Geometry check sheet. Reference: the model listing, model coordinates, mm. Face numbers are marked on the shaded views. A direction names the side the tool comes from. Round coordinates to 2 decimals unless told otherwise and drop trailing zeros. Write each loop counter-clockwise with the first axis right and the second up, starting at its lowest first coordinate (ties: lowest second). Pieces come first, ordered by that corner, then holes. Notation, with made-up numbers: M -2.5,-3.75 L 17.5,-3.75 A9 cw 17.5,3.25 Z; hole C 7.25,13 d6. An arc over 180 degrees is marked long. One line per item, written item: value. Start each with the question number.
1. Section check C-C (x = 0). Record the boundary of the cut face in (y, z).
2. Section check D-D (z = -11). Record the boundary of the cut face in (x, y), and give its area (3 significant figures).
3. Scan lines: probe 1 along Z at (x, y) = (0, 0.4); probe 2 along Y at (x, z) = (0, -6); probe 3 along X at (y, z) = (-17.5, 3). Record each from-to range of solid material in increasing order. Write a range as [from, to].
4. Release check for a two-part mould opening along X. For the marked faces 3, 4, 5 and 6 record: pulls with the +X half, pulls with the -X half, needs draft (parallel to the pull), parting line crosses it, or undercut.
5. Section check A-A (z = -16.5). Record the boundary of the cut face in (x, y).
6. Depth check by flat-ended pin: P1, Ø1.6, axis at y = 0.5, z = 20, coming from the +X side; P2, Ø1.5, axis at y = -20.5, z = 2.5, coming from the -X side; P3, Ø1.2, axis at x = 7.5, z = -4.5, coming from the -Y side. Enter the tip coordinate at first touch or a pass-through.
7. Section check B-B (y = -8.75). Record the boundary of the cut face in (x, z), and give its area (3 significant figures).
8. Access from +Z, -Z, +X, -X, +Y, -Y to the whole of each face (thin tool, end or side, straight path). Record for the marked faces 1 and 2.
Autodesk Inventor part; units mm, degrees
ref_plane "YZ Plane" through (0, 0, 0) normal (1, 0, 0) x (0, 1, 0)
ref_plane "XZ Plane" through (0, 0, 0) normal (0, 1, 0) x (-1, 0, 0)
ref_plane "XY Plane" through (0, 0, 0) normal (0, 0, 1) x (1, 0, 0)
sketch "Sketch1" plane through (0, 0, 0) normal (0, 1, 0) x (-1, 0, 0)
  line L0 (5, 25) -> (-5, 25)
  line L1 (-5, 25) -> (-5, -25)
  line L2 (-5, -25) -> (5, -25)
  line L3 (5, -25) -> (5, 25)
  line L4 (5, 25) -> (-5, -25) construction
  line L5 (-5, 25) -> (5, -25) construction
  circle A0 centre (0, 15) radius 2.5
  circle A1 centre (0, -15) radius 2.5
  point P0 (0, 0)
  point P1 (0, 25)
  dimension "d0" = 10
  dimension "d1" = 50
  dimension "d2" = 5
  dimension "d3" = 5
  dimension "d4" = 30
  dimension "d5" = 10
  dimension "d6" = 5
  dimension "d7" = 5
extrude "Extrusion1" add sketch "Sketch1" along normal blind 2
sketch "Sketch2" plane through (0, 0, 0) normal (0, -1, 0) x (1, 0, 0)
  line L0 (-5, -15) -> (-9, -15)
  line L1 (-5, 15) -> (-5.5, 15)
  circle A0 centre (0, -15) radius 2.5
  circle A1 centre (0, 15) radius 2.5
  arc A2 (-5.5, 15) -> (-9, -15) centre (110.994, -13.7951) ccw
  line L2 (-5, -15) -> (-5, 15)
  line L3 (-5, -25) -> (-5, 25)
  point P0 (0, 0)
  point P1 (-4, -14.9499)
  point P2 (-3, -15)
  dimension "d10" = 0
  dimension "d11" = 0
  dimension "d12" = 4
  dimension "d13" = 0.5
  dimension "d14" = 120
  dimension "d15" = 0
  dimension "d16" = 0
  dimension "d17" = 0
extrude "Extrusion2" add sketch "Sketch2" along normal blind 25 and the other way blind 2 contours L0 A2 L1 L2
sketch "Sketch3" plane through (0, 2, 0) normal (0, 1, 0) x (1, 0, 0)
  line L0 (5, -25) -> (5, 25)
  line L1 (5, 15) -> (9, 15)
  line L2 (5, -15) -> (5.5, -15)
  line L3 (5, -15) -> (5, 15)
  circle A0 centre (0, 15) radius 2.5
  circle A1 centre (0, -15) radius 2.5
  arc A2 (5.5, -15) -> (9, 15) centre (-110.994, 13.7951) ccw
  point P0 (0, 0)
  dimension "d22" = 0
  dimension "d23" = 0
  dimension "d24" = 0.5
  dimension "d25" = 4
  dimension "d26" = 120
extrude "Extrusion3" add sketch "Sketch3" against normal blind 25 contours L0 L1 A2 L2
properties part number "squeezer"
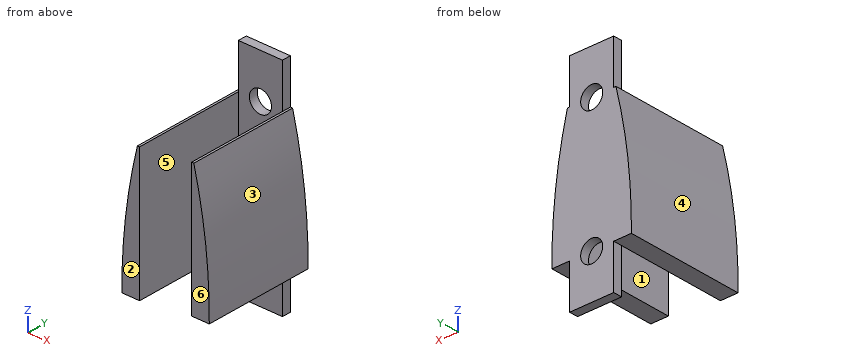
Result sheet:
1. outline: M 0,-25 L 2,-25 L 2,-17.5 L 0,-17.5 Z; M 0,-12.5 L 2,-12.5 L 2,12.5 L 0,12.5 Z; M 0,17.5 L 2,17.5 L 2,25 L 0,25 Z
2. outline: M -8.97,-25 L -5,-25 L -5,0 L 5,0 L 5,-23 L 8.97,-23 L 8.97,2 L -8.97,2 Z
2. area: 227 mm2
3. probe 1: z = [-25, -17.5], [-12.5, 12.5], [17.5, 25]
3. probe 2: y = [0, 2]
3. probe 3: x = [-7.82, -5], [5, 7.82]
4. face 3: pulls with the +X half
4. face 4: pulls with the -X half
4. face 5: undercut
4. face 6: needs draft
5. outline: M -5,0 L -2,0 L -2,2 L -5,2 Z; M 2,0 L 5,0 L 5,2 L 2,2 Z
6. P1: stops at x = 5
6. P2: stops at x = -7.99
6. P3: stops at y = -23
7. outline: M -9,-15 L -5,-15 L -5,15 L -5.5,15 A120 ccw Z; M 5,-15 L 9,-15 A120 ccw 5.5,15 L 5,15 Z
7. area: 173 mm2
8. face 1: +Z, -Z, -Y
8. face 2: +Z, -Z, +X, -X, -Y
